Verification items for the finished model (mm, model axes). Face numbers are marked on the shaded views. A direction names the side the tool comes from. Coordinates: 2 decimals unless noted, no trailing zeros. Order: outer loops, then holes, each group sorted by start corner. A loop starts at its lowest first (then second) coordinate and runs counter-clockwise, first axis right, second up. Notation, with made-up numbers: (70.25, 56) -> (90.25, 56) arc R10 cw to (90.25, 64) -> close; hole circle Ø4 at (83, -5.75). An arc over 180 degrees is marked (long way). Use CSV: the item, a comma, the result in double quotes. Start each with the question number.
1) Sectioned sample at D-D on y = 20. Record the boundary of the cut face in (x, z), then the cut area to 3 significant figures.
2) Sectioned sample at B-B on y = 6.5. Record the boundary of the cut face in (x, z).
3) Tool access check on the marked faces 1, 2, 3 and 4. Record the directions out of +Z, -Z, +X, -X, +Y, -Y that give a thin tool (end or side, any length) a straight path to the whole face; none if there is none.
4) Release check for a two-part mould opening along Y. For the marked faces 5, 6 and 7 record: released by +Y, released by -Y, zero draft, split by the parting line, or undercut.
5) Sectioned sample at A-A on x = 25. Record the boundary of the cut face in (y, z), then the cut area to 3 significant figures.
6) Go/stop test with flat-tipped pins: pin 1 (5 mm diameter, centred on x = 36, y = 27, fed in from +Z); pin 2 (4.5 mm diameter, centred on x = -6, y = 0, fed in from -Z); pin 3 (1.5 mm diameter, centred on y = 3.5, z = 6.5, fed in from +X); pin 4 (1.5 mm diameter, centred on x = 11, z = 9, fed in from -Y). Record where each tip stops, or that it passes through.
7) Scan lines: line 1 along Y through (x, z) = (-6, 7.75); line 2 along Y through (x, z) = (25, 1.6); line 3 along X through (y, z) = (0, 9). Record each from-to range of solid material in increasing order.
8) Sectioned sample at C-C on x = 6.5. Record the boundary of the cut face in (y, z), then the cut area to 3 significant figures.
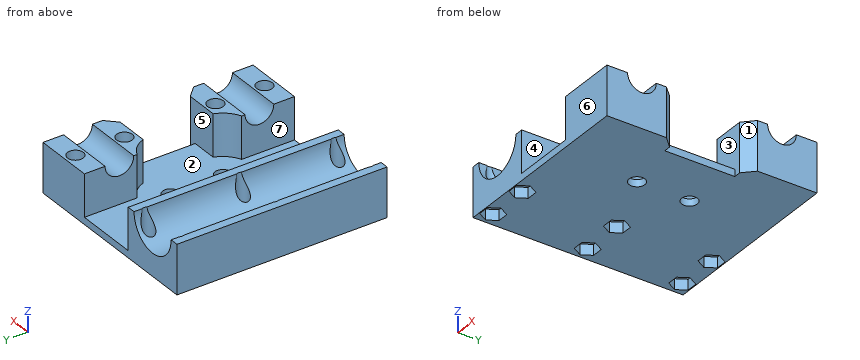
from build123d import *

# Parameters (mm, degrees)
SKETCH_W        = 55
SKETCH_H        = 60
PAD_DEPTH       = 14
SKETCH001_R     = 7.6
POCKET_DEPTH    = 60.001
SKETCH002_R     = 1.75
POCKET001_DEPTH = 14.001
POCKET002_DEPTH = 12
SKETCH004_R     = 2.25
POCKET003_DEPTH = 14.001
SKETCH008_R     = 4.1
POCKET005_DEPTH = 20
SKETCH010_W     = 20
SKETCH010_H     = 25
POCKET006_DEPTH = 5
SKETCH011_R     = 2.25
POCKET007_DEPTH = 10
CHAMFER_SIZE    = 3
CHAMFER001_SIZE = 3
POCKET008_DEPTH = 3


with BuildPart() as part:
    # Sketch → Pad (new body)
    with BuildSketch(Plane.XY):
        with Locations((17.5, 0)):
            Rectangle(SKETCH_W, SKETCH_H)
    extrude(amount=PAD_DEPTH)

    # Sketch001 → Pocket (cut, through all)
    with BuildSketch(Plane.XZ.offset(30)):
        with Locations((0, 14)):
            Circle(SKETCH001_R)
    extrude(amount=-POCKET_DEPTH, mode=Mode.SUBTRACT)

    # Sketch002 → Pocket001 (cut, through all)
    with BuildSketch(Plane(origin=(0, 0, 0), x_dir=(1, 0, 0), z_dir=(0, 0, -1))):
        with Locations((-6, 27)):
            Circle(SKETCH002_R)
        with Locations((-6, -27)):
            Circle(SKETCH002_R)
        with Locations((6, 27)):
            Circle(SKETCH002_R)
        with Locations((6, -27)):
            Circle(SKETCH002_R)
        with Locations((6, 0)):
            Circle(SKETCH002_R)
        with Locations((-6, 0)):
            Circle(SKETCH002_R)
    extrude(amount=-POCKET001_DEPTH, mode=Mode.SUBTRACT)

    # Sketch003 → Pocket002 (cut)
    with BuildSketch(Plane.XY.offset(14)):
        with BuildLine():
            Line((10, 35), (10, -35))
            Line((10, -35), (28, -35))
            Line((28, -35), (28, -14.916198))
            ThreePointArc((28, -14.916198), (30.841983, -12.965458), (32.599342, -10))
            Line((32.599342, -10), (52.599342, -10))
            Line((52.599342, -10), (52.599342, 10))
            Line((52.599342, 10), (32.599342, 10))
            ThreePointArc((32.599342, 10), (30.841983, 12.965458), (28, 14.916198))
            Line((28, 14.916198), (28, 35))
            Line((28, 35), (10, 35))
        make_face()
    extrude(amount=-POCKET002_DEPTH, mode=Mode.SUBTRACT)

    # Sketch004 → Pocket003 (cut, through all)
    with BuildSketch(Plane(origin=(0, 0, 0), x_dir=(1, 0, 0), z_dir=(0, 0, -1))):
        with Locations((25, 7.5)):
            Circle(SKETCH004_R)
        with Locations((25, -7.5)):
            Circle(SKETCH004_R)
    extrude(amount=-POCKET003_DEPTH, mode=Mode.SUBTRACT)

    # Sketch008 → Pocket005 (cut)
    with BuildSketch(Plane.YZ.offset(45)):
        with Locations((-20, 14)):
            Circle(SKETCH008_R)
        with Locations((20, 14)):
            Circle(SKETCH008_R)
    extrude(amount=-POCKET005_DEPTH, mode=Mode.SUBTRACT)

    # Sketch010 → Pocket006 (cut)
    with BuildSketch(Plane.YZ.offset(45)):
        with Locations((0, 6.5)):
            Rectangle(SKETCH010_W, SKETCH010_H)
    extrude(amount=-POCKET006_DEPTH, mode=Mode.SUBTRACT)

    # Sketch011 → Pocket007 (cut)
    with BuildSketch(Plane.XY.offset(14)):
        with Locations((36, 27)):
            Circle(SKETCH011_R)
        with Locations((36, 13)):
            Circle(SKETCH011_R)
        with Locations((36, -13)):
            Circle(SKETCH011_R)
        with Locations((36, -27)):
            Circle(SKETCH011_R)
    extrude(amount=-POCKET007_DEPTH, mode=Mode.SUBTRACT)

    # Chamfer
    chamfer_edges = [part.edges().sort_by_distance(p)[0] for p in [
        (45, -10, 8),
        (45, -10, 1),
    ]]
    chamfer(chamfer_edges, length=CHAMFER_SIZE)

    # Chamfer001
    chamfer001_edges = [part.edges().sort_by_distance(p)[0] for p in [
        (45, 10, 8),
        (45, 10, 1),
    ]]
    chamfer(chamfer001_edges, length=CHAMFER001_SIZE)

    # Sketch012 → Pocket008 (cut)
    with BuildSketch(Plane(origin=(0, 0, 0), x_dir=(1, 0, 0), z_dir=(0, 0, -1))):
        Polygon((-4.412285, 29.750003), (-7.587715, 29.750003), (-9.17543, 27), (-7.587715, 24.249997), (-4.412285, 24.249997), (-2.82457, 27), align=None)
        Polygon((7.587715, 29.750003), (4.412285, 29.750003), (2.82457, 27), (4.412285, 24.249997), (7.587715, 24.249997), (9.17543, 27), align=None)
        Polygon((-4.412285, 2.750003), (-7.587715, 2.750003), (-9.17543, 0), (-7.587715, -2.750003), (-4.412285, -2.750003), (-2.82457, 0), align=None)
        Polygon((7.587715, 2.750003), (4.412285, 2.750003), (2.82457, 0), (4.412285, -2.750003), (7.587715, -2.750003), (9.17543, 0), align=None)
        Polygon((-4.412285, -24.249997), (-7.587715, -24.249997), (-9.17543, -27), (-7.587715, -29.750003), (-4.412285, -29.750003), (-2.82457, -27), align=None)
        Polygon((7.587715, -24.249997), (4.412285, -24.249997), (2.82457, -27), (4.412285, -29.750003), (7.587715, -29.750003), (9.17543, -27), align=None)
    extrude(amount=-POCKET008_DEPTH, mode=Mode.SUBTRACT)


solid = part.part
Answers follow:
1,outline,"(-10, 0) -> (45, 0) -> (45, 9.9) -> (28, 9.9) -> (28, 2) -> (10, 2) -> (10, 14) -> (7.6, 14) arc R7.6 cw to (-7.6, 14) -> (-10, 14) -> close"
1,area,"394 mm²"
2,outline,"(-10, 0) -> (22.98, 0) -> (22.98, 2) -> (10, 2) -> (10, 14) -> (7.6, 14) arc R7.6 cw to (-7.6, 14) -> (-10, 14) -> close; (27.02, 0) -> (40, 0) -> (40, 2) -> (27.02, 2) -> close"
3,face 1,"+Z, -Z, +X"
3,face 2,"+Z"
3,face 3,"+Z, +X"
3,face 4,"+Z, +Y, -Y"
4,face 5,"undercut"
4,face 6,"released by -Y"
4,face 7,"zero draft"
5,outline,"(-30, 0) -> (-9.75, 0) -> (-9.75, 2) -> (-30, 2) -> close; (-5.25, 0) -> (5.25, 0) -> (5.25, 2) -> (-5.25, 2) -> close; (9.75, 0) -> (30, 0) -> (30, 2) -> (9.75, 2) -> close"
5,area,"102 mm²"
6,pin 1,"stops at z = 14"
6,pin 2,"stops at z = 3"
6,pin 3,"stops at x = 10"
6,pin 4,"passes through"
7,line 1,"y = -30 to -28.75, -25.25 to -1.75, 1.75 to 25.25, 28.75 to 30"
7,line 2,"y = -30 to -9.75, -5.25 to 5.25, 9.75 to 30"
7,line 3,"x = -10 to -7.75, 7.75 to 10"
8,outline,"(-30, 0) -> (-29.75, 0) -> (-29.75, 3) -> (-28.68, 3) -> (-28.68, 10.06) -> (-30, 10.06) -> close; (-25.32, 3) -> (-24.25, 3) -> (-24.25, 0) -> (-2.75, 0) -> (-2.75, 3) -> (-1.68, 3) -> (-1.68, 10.06) -> (-25.32, 10.06) -> close; (1.68, 3) -> (2.75, 3) -> (2.75, 0) -> (24.25, 0) -> (24.25, 3) -> (25.32, 3) -> (25.32, 10.06) -> (1.68, 10.06) -> close; (28.68, 3) -> (29.75, 3) -> (29.75, 0) -> (30, 0) -> (30, 10.06) -> (28.68, 10.06) -> close"
8,area,"483 mm²"
